from build123d import *

# Parameters (mm, degrees)
SKETCH1_R           = 19.05
BOSS_EXTRUDE1_DEPTH = 1.5875
SKETCH2_R           = 16.1671
BOSS_EXTRUDE2_DEPTH = 12.7
SKETCH3_R           = 19.05
BOSS_EXTRUDE3_DEPTH = 1.5875
SKETCH4_R           = 11.1125
BOSS_EXTRUDE4_DEPTH = 6.35
CUT_EXTRUDE1_REACH  = 36.925
SKETCH5_R           = 3.175


with BuildPart() as part:
    # Sketch1 → Boss-Extrude1 (new body)
    with BuildSketch(Plane(origin=(0, 0, 0), x_dir=(1, 0, 0), z_dir=(0, 1, 0))):
        with Locations(Location((0, 0, 0), (0, 0, 270))):
            Circle(SKETCH1_R)
    extrude(amount=BOSS_EXTRUDE1_DEPTH)

    # Sketch2 → Boss-Extrude2 (add)
    with BuildSketch(Plane(origin=(0, 1.5875, 0), x_dir=(1, 0, 0), z_dir=(0, 1, 0))):
        with Locations(Location((0, 0, 0), (0, 0, 270))):
            Circle(SKETCH2_R)
    extrude(amount=BOSS_EXTRUDE2_DEPTH)

    # Sketch3 → Boss-Extrude3 (add)
    with BuildSketch(Plane(origin=(0, 14.2875, 0), x_dir=(1, 0, 0), z_dir=(0, 1, 0))):
        with Locations(Location((0, 0, 0), (0, 0, 270))):
            Circle(SKETCH3_R)
    extrude(amount=BOSS_EXTRUDE3_DEPTH)

    # Sketch4 → Boss-Extrude4 (add)
    with BuildSketch(Plane(origin=(0, 15.875, 0), x_dir=(1, 0, 0), z_dir=(0, 1, 0))):
        with Locations(Location((0, 0, 0), (0, 0, 270))):
            Circle(SKETCH4_R)
    extrude(amount=BOSS_EXTRUDE4_DEPTH)

    # Sketch5 → Cut-Extrude1 (cut, up to next)
    with BuildSketch(Plane(origin=(0, 22.225, 0), x_dir=(1, 0, 0), z_dir=(0, 1, 0)), mode=Mode.PRIVATE) as cut_extrude1_sk1:
        with Locations(Location((0, 0, 0), (0, 0, 270))):
            Circle(SKETCH5_R)
    cut_extrude1_tool1 = extrude(cut_extrude1_sk1.sketch, amount=-CUT_EXTRUDE1_REACH, mode=Mode.PRIVATE) & part.part
    add(cut_extrude1_tool1.solids().sort_by_distance((0, 22.225, 0))[0], mode=Mode.SUBTRACT)


solid = part.part
The listing builds one solid part. Answer for the finished solid, in the listing's coordinates (mm). A direction names the side the tool comes from. Give positions to 0.01 mm unless a question says otherwise; leave off trailing zeros. Write each loop counter-clockwise with the first axis right and the second up, starting at its lowest first coordinate (ties: lowest second). Pieces come first, ordered by that corner, then holes.
Item 1: Determine the mould class of faces 1 (the cylindrical face through (-11.59, 0.78, -15.12)), 2 (the cylindrical face through (-1.93, 11.27, -2.52)), 3 (the flat face through (-14, 14.288, -9)) for opening direction X: released by +X, released by -X, zero draft, split by the parting line, or undercut.
Item 2: Section D-D, the plane x = -14.5 is taken. Write down the section's boundary in (y, z) (1 decimal), plus the area to 3 significant figures.
Item 3: Find the intervals of material crossed by line 1 along X through (y, z) = (7.25, 0) (3 decimals); line 2 along Y through (x, z) = (7, 16.5) (1 decimal); line 3 along X through (y, z) = (15.75, 0) (3 decimals), in increasing order.
Item 4: Section C-C, the plane y = 5.75 is taken. Write down the section's boundary in (x, z) (3 decimals).
Item 5: Flat-ended cylindrical pins translate along their axes: P1, Ø2, axis at y = 16, z = -14, coming from the -X side; P2, Ø5, axis at x = 11.5, y = 7.5, coming from the -Z side; P3, Ø10, axis at x = -11.5, y = 18, coming from the -Z side. Find the tip coordinate at first contact, or state that the pin passes through.
Item 6: Which of the six approach directions +Z, -Z, +X, -X, +Y, -Y give full straight-line access (tool end or side, diameter ignored) to faces 4 (the flat face through (-8, 15.875, 8)), 5 (the cylindrical face through (16.03, 7.85, -2.1)), 6 (the flat face through (0, 0, 4))?
Completed:
1. face 1: split by the parting line
1. face 2: undercut
1. face 3: zero draft
2. outline: (0, -12.4) - (1.6, -12.4) - (1.6, -7.2) - (14.3, -7.2) - (14.3, -12.4) - (15.9, -12.4) - (15.9, 12.4) - (14.3, 12.4) - (14.3, 7.2) - (1.6, 7.2) - (1.6, 12.4) - (0, 12.4) - close
2. area: 260 mm2
3. line 1: x = -16.167 to -3.175, 3.175 to 16.167
3. line 2: y = 0 to 1.6, 14.3 to 15.9
3. line 3: x = -19.05 to -3.175, 3.175 to 19.05
4. outline: circle Ø32.334 at (0, 0); hole circle Ø6.35 at (0, 0)
5. P1: stops at x = -13.92
5. P2: stops at z = -13.43
5. P3: stops at z = -17.73
6. face 4: +Y
6. face 5: none
6. face 6: +Z, -Z, +X, -X, -Y
